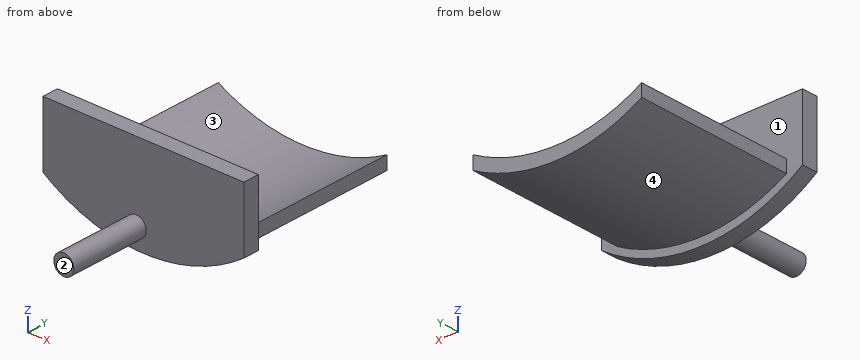
```python
from build123d import *

# Parameters (mm, degrees)
BOSS_EXTRUDE1_DEPTH = 2.54
BOSS_EXTRUDE2_DEPTH = 25.4
SKETCH4_W           = 31.75
SKETCH4_H           = 16.51
CUT_EXTRUDE1_DEPTH  = 2.54
SKETCH5_R           = 1.5875
BOSS_EXTRUDE3_DEPTH = 12.7


with BuildPart() as part:
    # Sketch1 → Boss-Extrude1 (new body)
    with BuildSketch(Plane(origin=(0, 0, 0), x_dir=(1, 0, 0), z_dir=(0, 1, 0))):
        with BuildLine():
            Line((0, 0), (31.75, 0))
            Line((31.75, 0), (31.75, 26.649569904))
            ThreePointArc((31.75, 26.649569904), (15.875, 31.75), (0, 26.649569904))
            Line((0, 26.649569904), (0, 0))
        make_face()
    extrude(amount=BOSS_EXTRUDE1_DEPTH)

    # Sketch2 → Boss-Extrude2 (add)
    with BuildSketch(Plane(origin=(0, 2.54, 0), x_dir=(1, 0, 0), z_dir=(0, 1, 0))):
        with BuildLine():
            Line((2.54, 26.911706478), (2.54, 24.951669261))
            ThreePointArc((2.54, 24.951669261), (15.875, 28.448), (29.21, 24.951669261))
            Line((29.21, 24.951669261), (29.21, 27.054735))
            ThreePointArc((29.21, 27.054735), (15.856249221, 30.479609179), (2.54, 26.911706478))
        make_face()
    extrude(amount=BOSS_EXTRUDE2_DEPTH)

    # Sketch4 → Cut-Extrude1 (cut)
    with BuildSketch(Plane.XZ):
        with Locations((15.875, -8.255)):
            Rectangle(SKETCH4_W, SKETCH4_H)
    extrude(amount=-CUT_EXTRUDE1_DEPTH, mode=Mode.SUBTRACT)

    # Sketch5 → Boss-Extrude3 (add)
    with BuildSketch(Plane.XZ):
        with Locations((14.732, -28.575)):
            Circle(SKETCH5_R)
    extrude(amount=BOSS_EXTRUDE3_DEPTH)


solid = part.part
```
The listing builds one solid part. Answer for the finished solid, in the listing's coordinates (mm). Face numbers are marked on the shaded views. Round coordinates to 2 decimals unless told otherwise and drop trailing zeros. Loops run counter-clockwise (first coordinate to the right, second up) from the corner with the lowest first, then second, coordinate; pieces in that order, holes last. Notation, with made-up numbers: (-22.5, -25) -> (5.5, -25) arc R19 ccw to (5.5, -7) -> close; hole circle Ø6 at (69.25, 23). An arc over 180 degrees is marked (long way). Use one line per item in the form item = value.
1. The part is cut by section B-B on z = -19. Determine the outline of the cut face in (x, y).
Answer key:
outline = (0, 0) -> (31.75, 0) -> (31.75, 2.54) -> (0, 2.54) -> close
2. The part is cut by section C-C on y = 17.5. Determine the outline of the cut face in (x, z) (3 decimals).
Answer key:
outline = (2.54, -26.912) arc R27.178 ccw to (29.21, -27.055) -> (29.21, -24.952) arc R27.178 cw to (2.54, -24.952) -> close
3. Find the intervals of material crossed by probe 1 along Y at (x, z) = (12, -23); probe 2 along X at (y, z) = (7, -25.75); probe 3 along X at (y, z) = (5, -25.25), in increasing order. Write a range as [from, to].
Answer key:
probe_1 = [0, 2.54]
probe_2 = [2.54, 4.07], [27.68, 29.21]
probe_3 = [2.54, 3.08], [28.67, 29.21]
4. Flat-ended cylindrical pins translate along their axes: pin 1 Ø2.5 at (y, z) = (20, -26) entering from +X; pin 2 Ø1.5 at (x, z) = (7, -21.5) entering from -Y; pin 3 Ø4 at (x, y) = (20.5, 12) entering from -Z. Find the tip coordinate at first contact, or state that the pin passes through.
Answer key:
pin_1 = 29.21
pin_2 = 0
pin_3 = -30.36
5. The part is cut by section D-D on z = -26. Determine the outline of the cut face in (x, y), and give its area (3 significant figures).
Answer key:
outline = (0, 0) -> (31.75, 0) -> (31.75, 2.54) -> (29.21, 2.54) -> (29.21, 27.94) -> (27.15, 27.94) -> (27.15, 2.54) -> (4.6, 2.54) -> (4.6, 27.94) -> (2.54, 27.94) -> (2.54, 2.54) -> (0, 2.54) -> close
area = 185 mm²
6. The part is cut by section A-A on x = 6. Determine the outline of the cut face in (y, z).
Answer key:
outline = (0, -29.9) -> (2.54, -29.9) -> (2.54, -28.57) -> (27.94, -28.57) -> (27.94, -26.59) -> (2.54, -26.59) -> (2.54, -16.51) -> (0, -16.51) -> close
7. For a pull along X with two mould halves and no side action, classify the marked faces 1, 2, 3 and 4 as released by +X, released by -X, zero draft, split by the parting line, or undercut.
Answer key:
face_1 = undercut
face_2 = zero draft
face_3 = undercut
face_4 = split by the parting line
